```python
from build123d import *

# Parameters (mm, degrees)
SKETCH_1_R          = 2
EXTRUDE_1_DEPTH     = 5
SKETCH_2_R          = 1.5
CUT_EXTRUDE_1_DEPTH = 129.986884904
CUT_EXTRUDE_2_DEPTH = 3
CUT_EXTRUDE_3_DEPTH = 3
CUT_EXTRUDE_4_DEPTH = 129.986884904
FILLET_1_R          = 10
FILLET_2_R          = 10
FILLET_3_R          = 10
CUT_EXTRUDE_6_DEPTH = 127.770989194
FILLET_4_R          = 3
SKETCH_8_R          = 1.5
CUT_EXTRUDE_7_DEPTH = 127.770989194
SKETCH_9_R          = 1.25
CUT_EXTRUDE_8_DEPTH = 127.770989194
SKETCH_10_R         = 1.5
CUT_EXTRUDE_9_DEPTH = 127.770989194


with BuildPart() as part:
    # 草图1 → 凸台-拉伸1 (new body)
    # profile 1 of 3: a face of its own
    with BuildSketch(Plane(origin=(0, 0, 0), x_dir=(1, 0, 0), z_dir=(0, 1, 0))):
        with BuildLine():
            ThreePointArc((90, 50.256494602), (0, 40), (-90, 50.256494602))
            Line((-90, 50.256494602), (-90, -65))
            Line((-90, -65), (90, -65))
            Line((90, -65), (90, 50.256494602))
        make_face()
        with Locations(Location((-72, -8.5, 0), (0, 0, 270))):
            Circle(SKETCH_1_R, mode=Mode.SUBTRACT)
        with Locations(Location((72, -8.5, 0), (0, 0, 270))):
            Circle(SKETCH_1_R, mode=Mode.SUBTRACT)
    # profile 2 of 3: a face of its own
    with BuildSketch(Plane(origin=(0, 0, 0), x_dir=(1, 0, 0), z_dir=(0, 1, 0))):
        with BuildLine():
            Line((-90, -65), (-90, 50.256494602))
            ThreePointArc((-90, 50.256494602), (-100.687943549, 52.879943656), (-111.299669708, 55.796429581))
            Line((-111.299669708, 55.796429581), (-90, -65))
        make_face()
    # profile 3 of 3: a face of its own
    with BuildSketch(Plane(origin=(0, 0, 0), x_dir=(1, 0, 0), z_dir=(0, 1, 0))):
        with BuildLine():
            ThreePointArc((111.299669708, 55.796429581), (100.687943549, 52.879943656), (90, 50.256494602))
            Line((90, 50.256494602), (90, -65))
            Line((90, -65), (111.299669708, 55.796429581))
        make_face()
    extrude(amount=EXTRUDE_1_DEPTH)

    # 草图2 → 切除-拉伸1 (cut, through all)
    with BuildSketch(Plane(origin=(0, 0, 0), x_dir=(-1, 0, 0), z_dir=(0, -1, 0))):
        with Locations(Location((6, 18.25, 0), (0, 0, 90))):
            Circle(SKETCH_2_R)
        with Locations(Location((-6, 18.25, 0), (0, 0, 90))):
            Circle(SKETCH_2_R)
        with Locations(Location((6, 24.75, 0), (0, 0, 90))):
            Circle(SKETCH_2_R)
        with Locations(Location((-6, 24.75, 0), (0, 0, 90))):
            Circle(SKETCH_2_R)
        with Locations(Location((-6, 34.75, 0), (0, 0, 90))):
            Circle(SKETCH_2_R)
        with Locations(Location((6, 34.75, 0), (0, 0, 90))):
            Circle(SKETCH_2_R)
    extrude(amount=-CUT_EXTRUDE_1_DEPTH, mode=Mode.SUBTRACT)

    # 草图3 → 切除-拉伸2 (cut)
    with BuildSketch(Plane(origin=(0, 5, 0), x_dir=(1, 0, 0), z_dir=(0, 1, 0))):
        with BuildLine():
            ThreePointArc((-45, -46.5), (-40, -41.5), (-35, -46.5))
            Line((-35, -46.5), (-35, 8.5))
            ThreePointArc((-35, 8.5), (-40, 3.5), (-45, 8.5))
            Line((-45, 8.5), (-45, -46.5))
        make_face()
        with BuildLine():
            ThreePointArc((-45, 8.5), (-40, 3.5), (-35, 8.5))
            Line((-35, 8.5), (-45, 8.5))
        make_face()
        with BuildLine():
            Line((-45, 8.5), (-35, 8.5))
            ThreePointArc((-35, 8.5), (-40, 13.5), (-45, 8.5))
        make_face()
        with BuildLine():
            ThreePointArc((-45, -46.5), (-40, -51.5), (-35, -46.5))
            Line((-35, -46.5), (-45, -46.5))
        make_face()
        with BuildLine():
            Line((-45, -46.5), (-35, -46.5))
            ThreePointArc((-35, -46.5), (-40, -41.5), (-45, -46.5))
        make_face()
        with BuildLine():
            ThreePointArc((45, 8.5), (40, 3.5), (35, 8.5))
            Line((35, 8.5), (35, -46.5))
            ThreePointArc((35, -46.5), (40, -41.5), (45, -46.5))
            Line((45, -46.5), (45, 8.5))
        make_face()
        with BuildLine():
            ThreePointArc((45, -46.5), (40, -41.5), (35, -46.5))
            Line((35, -46.5), (45, -46.5))
        make_face()
        with BuildLine():
            Line((45, -46.5), (35, -46.5))
            ThreePointArc((35, -46.5), (40, -51.5), (45, -46.5))
        make_face()
        with BuildLine():
            ThreePointArc((45, 8.5), (40, 13.5), (35, 8.5))
            Line((35, 8.5), (45, 8.5))
        make_face()
        with BuildLine():
            Line((45, 8.5), (35, 8.5))
            ThreePointArc((35, 8.5), (40, 3.5), (45, 8.5))
        make_face()
    extrude(amount=-CUT_EXTRUDE_2_DEPTH, mode=Mode.SUBTRACT)

    # 草图4 → 切除-拉伸3 (cut)
    with BuildSketch(Plane(origin=(0, 5, 0), x_dir=(1, 0, 0), z_dir=(0, 1, 0))):
        with BuildLine():
            Line((45, -41.966401061), (45, -27.473665961))
            ThreePointArc((45, -27.473665961), (39.285969894, -12.835001066), (40.990143514, 2.78666473))
            Line((40.990143514, 2.78666473), (35, 4.966898668))
            Line((35, 4.966898668), (35, -30.4089023))
            ThreePointArc((35, -30.4089023), (39.482405618, -36.635494586), (45, -41.966401061))
        make_face()
        with BuildLine():
            Line((35, 4.966898668), (31.593217306, 6.206866163))
            ThreePointArc((31.593217306, 6.206866163), (29.1849194, -12.483575431), (35, -30.4089023))
            Line((35, -30.4089023), (35, 4.966898668))
        make_face()
        with BuildLine():
            Line((72, -51.5), (72, -41.5))
            ThreePointArc((72, -41.5), (56.787028178, -37.784219101), (45, -27.473665961))
            Line((45, -27.473665961), (45, -41.966401061))
            ThreePointArc((45, -41.966401061), (57.6831436, -49.046610497), (72, -51.5))
        make_face()
    extrude(amount=-CUT_EXTRUDE_3_DEPTH, mode=Mode.SUBTRACT)

    # 草图5 → 切除-拉伸4 (cut, through all)
    with BuildSketch(Plane(origin=(0, 5, 0), x_dir=(1, 0, 0), z_dir=(0, 1, 0))):
        Polygon((23, 15), (23, -55), (88, -55), (51, 15), align=None)
        Polygon((-88, -55), (-51, 15), (-23, 15), (-23, -55), align=None)
    extrude(amount=-CUT_EXTRUDE_4_DEPTH, mode=Mode.SUBTRACT)

    # 圆角1
    fillet_1_edges = [part.edges().sort_by_distance(p)[0] for p in [
        (23, 2.5, -15),
        (51, 2.5, -15),
        (88, 2.5, 55),
        (23, 2.5, 55),
        (-23, 2.5, 55),
        (-88, 2.5, 55),
        (-51, 2.5, -15),
        (-23, 2.5, -15),
    ]]
    fillet(fillet_1_edges, radius=FILLET_1_R)

    # 圆角2
    fillet_2_edges = [part.edges().sort_by_distance(p)[0] for p in [
        (90, 2.5, 65),
        (-90, 2.5, 65),
    ]]
    fillet(fillet_2_edges, radius=FILLET_2_R)

    # 圆角3
    fillet_3_edges = [part.edges().sort_by_distance(p)[0] for p in [
        (111.299669708, 2.5, -55.796429581),
        (-111.299669708, 2.5, -55.796429581),
    ]]
    fillet(fillet_3_edges, radius=FILLET_3_R)

    # 草图7 → 切除-拉伸6 (cut, through all)
    with BuildSketch(Plane(origin=(0, 5, 0), x_dir=(1, 0, 0), z_dir=(0, 1, 0))):
        Polygon((-65, 30), (-84.345864805, -6.600284766), (-92.1600328, 37.716064119), align=None)
        Polygon((84.345864805, -6.600284766), (92.1600328, 37.716064119), (65, 30), align=None)
    extrude(amount=-CUT_EXTRUDE_6_DEPTH, mode=Mode.SUBTRACT)

    # 圆角4
    fillet_4_edges = [part.edges().sort_by_distance(p)[0] for p in [
        (-92.1600328, 2.5, -37.716064119),
        (-65, 2.5, -30),
        (-84.345864805, 2.5, 6.600284766),
        (84.345864805, 2.5, 6.600284766),
        (65, 2.5, -30),
        (92.1600328, 2.5, -37.716064119),
    ]]
    fillet(fillet_4_edges, radius=FILLET_4_R)

    # 草图8 → 切除-拉伸7 (cut, through all)
    with BuildSketch(Plane(origin=(0, 0, 0), x_dir=(-1, 0, 0), z_dir=(0, -1, 0))):
        with Locations(Location((-55.513531222, 30, 0), (0, 0, 90))):
            Circle(SKETCH_8_R)
        with Locations(Location((-86.847160275, -25, 0), (0, 0, 90))):
            Circle(SKETCH_8_R)
        with Locations(Location((55.513531222, 30, 0), (0, 0, 90))):
            Circle(SKETCH_8_R)
        with Locations(Location((86.847160275, -25, 0), (0, 0, 90))):
            Circle(SKETCH_8_R)
    extrude(amount=-CUT_EXTRUDE_7_DEPTH, mode=Mode.SUBTRACT)

    # 草图9 → 切除-拉伸8 (cut, through all)
    with BuildSketch(Plane.XZ):
        with Locations(Location((0, -14, 0), (0, 0, 270))):
            Circle(SKETCH_9_R)
        with Locations(Location((0, -6.5, 0), (0, 0, 270))):
            Circle(SKETCH_9_R)
        with Locations(Location((0, 1, 0), (0, 0, 270))):
            Circle(SKETCH_9_R)
        with Locations(Location((0, 8.5, 0), (0, 0, 270))):
            Circle(SKETCH_9_R)
        with Locations(Location((0, 16, 0), (0, 0, 270))):
            Circle(SKETCH_9_R)
        with Locations(Location((0, 23.5, 0), (0, 0, 270))):
            Circle(SKETCH_9_R)
        with Locations(Location((0, 31, 0), (0, 0, 270))):
            Circle(SKETCH_9_R)
        with Locations(Location((0, 38.5, 0), (0, 0, 270))):
            Circle(SKETCH_9_R)
        with Locations(Location((0, 46, 0), (0, 0, 270))):
            Circle(SKETCH_9_R)
        with Locations(Location((0, 53.5, 0), (0, 0, 270))):
            Circle(SKETCH_9_R)
        with Locations(Location((0, 61, 0), (0, 0, 270))):
            Circle(SKETCH_9_R)
    extrude(amount=-CUT_EXTRUDE_8_DEPTH, mode=Mode.SUBTRACT)

    # 草图10 → 切除-拉伸9 (cut, through all)
    with BuildSketch(Plane.XZ):
        with Locations(Location((-15, 25, 0), (0, 0, 270))):
            Circle(SKETCH_10_R)
        with Locations(Location((-15, 5, 0), (0, 0, 270))):
            Circle(SKETCH_10_R)
        with Locations(Location((15, 5, 0), (0, 0, 90))):
            Circle(SKETCH_10_R)
        with Locations(Location((15, 25, 0), (0, 0, 90))):
            Circle(SKETCH_10_R)
    extrude(amount=-CUT_EXTRUDE_9_DEPTH, mode=Mode.SUBTRACT)


solid = part.part
```
Can you work these out from the model? Positions are in its coordinate system, mm. A direction names the side the tool comes from. Coordinates: 2 decimals unless noted, no trailing zeros. Loops run counter-clockwise (first coordinate to the right, second up) from the corner with the lowest first, then second, coordinate; pieces in that order, holes last.
1) For pin 1 (1.5 mm diameter, centred on x = 67, z = 12, fed in from -Y); pin 2 (1.5 mm diameter, centred on y = 3.5, z = 12.5, fed in from -X), each with a flat end and sliding along its axis, tell me the tip position at first contact or that it passes through.
2) Imagine slicing it at C-C on x = -39. List the corners of the cut face in (y, z) for me, plus the area to 3 significant figures.
3) Which directions (+Z, -Z, +X, -X, +Y, -Y) give clear straight access to the entire face, cutting with the end or side of a thin tool? Please do faces 1 (the flat face through (-52, 3, 55)), 2 (the flat face through (-1, 2, 65)).
4) Imagine slicing it at A-A on z = -44.5. List the corners of the cut face in (x, y) for me.
5) I need wall thicknesses on probe 1 along X at (y, z) = (4.3, -16); probe 2 along Z at (x, y) = (76, 4.4); probe 3 along Z at (x, y) = (-68, 4.45). Which ranges of each line are inside material? Lowest first, please.
6) Thinking about a two-plate mould opening in X: for faces 3 (the flat face through (-88.56, 2.54, -17.29)), 4 (the cylindrical face through (88.11, 2.54, 62.6)), 5 (the flat face through (-100.134, 2.465, 7.525)), which applies, pulls with the +X half, pulls with the -X half, needs draft (parallel to the pull), parting line crosses it, or undercut?
7) Imagine slicing it at B-B on x = 76.5. List the corners of the cut face in (y, z) for me, plus the area to 3 significant figures.
8) Imagine slicing it at D-D on y = 3. State how many separate pieces and enclosed holes the cut face has, plus the area to 3 significant figures.
Completed:
1. pin 1: stops at y = 0
1. pin 2: stops at x = -99.39
2. outline: (0, -41.91) - (5, -41.91) - (5, -15) - (0, -15) - close; (0, 55) - (5, 55) - (5, 65) - (0, 65) - close
2. area: 185 mm2
3. face 1: +Y, -Y
3. face 2: +Z, +X, -X, +Y, -Y
4. outline: (-108.42, 0) - (-59.83, 0) - (-59.83, 5) - (-108.42, 5) - close; (59.83, 0) - (108.42, 0) - (108.42, 5) - (59.83, 5) - close
5. probe 1: x = -104.28 to -88.33, -72.4 to 72.4, 88.33 to 104.28
5. probe 2: z = -47.29 to -33.13, -9.19 to 32.3, 53.88 to 65
5. probe 3: z = -45.82 to -30.79, -24.32 to 17.16, 55 to 65
6. face 3: undercut
6. face 4: pulls with the +X half
6. face 5: pulls with the -X half
7. outline: (0, -47.38) - (5, -47.38) - (5, -33.27) - (0, -33.27) - close; (0, -8.24) - (5, -8.24) - (5, 33.24) - (0, 33.24) - close; (0, 53.6) - (5, 53.6) - (5, 65) - (0, 65) - close
7. area: 335 mm2
8. separate pieces: 1
8. enclosed holes: 31
8. area: 14,300 mm2
